```python
from build123d import *

# Parameters (mm, degrees)
SKETCH1_W           = 60
SKETCH1_H           = 40
BOSS_EXTRUDE1_DEPTH = 10
BOSS_EXTRUDE2_START = 5
SKETCH2_R           = 2.5
BOSS_EXTRUDE2_DEPTH = 5
BOSS_EXTRUDE3_START = -10
SKETCH2_3_R         = 2.5
BOSS_EXTRUDE3_DEPTH = 5
SKETCH3_W           = 34
SKETCH3_H           = 4
CUT_EXTRUDE1_DEPTH  = 124.434192994


with BuildPart() as part:
    # Sketch1 → Boss-Extrude1 (new body)
    with BuildSketch(Plane(origin=(0, 0, 0), x_dir=(1, 0, 0), z_dir=(0, 1, 0))):
        Rectangle(SKETCH1_W, SKETCH1_H)
    extrude(amount=BOSS_EXTRUDE1_DEPTH)

    # Sketch2 → Boss-Extrude2 (add)
    with BuildSketch(Plane(origin=(0, 0, 0), x_dir=(0, 0, -1), z_dir=(1, 0, 0)).offset(BOSS_EXTRUDE2_START)):
        with BuildLine():
            Line((20, 10), (20, 100))
            ThreePointArc((20, 100), (14, 106), (8, 100))
            Line((8, 100), (-20, 10))
            Line((-20, 10), (20, 10))
        make_face()
        with Locations((14, 25)):
            Circle(SKETCH2_R, mode=Mode.SUBTRACT)
        with Locations((14, 50)):
            Circle(SKETCH2_R, mode=Mode.SUBTRACT)
        with Locations((14, 75)):
            Circle(SKETCH2_R, mode=Mode.SUBTRACT)
        with Locations((14, 100)):
            Circle(SKETCH2_R, mode=Mode.SUBTRACT)
    extrude(amount=BOSS_EXTRUDE2_DEPTH)

    # Sketch2<3> → Boss-Extrude3 (add)
    with BuildSketch(Plane(origin=(0, 0, 0), x_dir=(0, 0, -1), z_dir=(1, 0, 0)).offset(BOSS_EXTRUDE3_START)):
        with BuildLine():
            Line((20, 10), (20, 100))
            ThreePointArc((20, 100), (14, 106), (8, 100))
            Line((8, 100), (-20, 10))
            Line((-20, 10), (20, 10))
        make_face()
        with Locations((14, 25)):
            Circle(SKETCH2_3_R, mode=Mode.SUBTRACT)
        with Locations((14, 50)):
            Circle(SKETCH2_3_R, mode=Mode.SUBTRACT)
        with Locations((14, 75)):
            Circle(SKETCH2_3_R, mode=Mode.SUBTRACT)
        with Locations((14, 100)):
            Circle(SKETCH2_3_R, mode=Mode.SUBTRACT)
    extrude(amount=BOSS_EXTRUDE3_DEPTH)

    # Sketch3 → Cut-Extrude1 (cut, through all)
    with BuildSketch(Plane.ZY.offset(30)):
        with Locations((0, 5)):
            Rectangle(SKETCH3_W, SKETCH3_H)
    extrude(amount=-CUT_EXTRUDE1_DEPTH, mode=Mode.SUBTRACT)


solid = part.part
```
The model under review builds one solid part; all positions refer to its coordinate system, in mm. A direction names the side the tool comes from. Round coordinates to 2 decimals unless told otherwise and drop trailing zeros. Order: outer loops, then holes, each group sorted by start corner. A loop starts at its lowest first (then second) coordinate and runs counter-clockwise, first axis right, second up. Notation, with made-up numbers: M -20,17 L -3,17 A22 ccw -3,44 Z; hole C 57.25,-30 d5. An arc over 180 degrees is marked long. Use a Markdown table: item, result.
1) Consider section A-A (y = 14.5). Write out the cut boundary in (x, z), then the cut area to 3 significant figures.
Report:
| item | result |
|---|---|
| outline | M -10,-20 L -5,-20 L -5,18.6 L -10,18.6 Z; M 5,-20 L 10,-20 L 10,18.6 L 5,18.6 Z |
| area | 386 mm^2 |
2) Consider section B-B (x = 7.5). Write out the cut boundary in (y, z).
Report:
| item | result |
|---|---|
| outline | M 0,-20 L 100,-20 A6 ccw 100,-8 L 10,20 L 0,20 Z; hole M 3,-17 L 7,-17 L 7,17 L 3,17 Z; hole C 25,-14 d5; hole C 50,-14 d5; hole C 75,-14 d5; hole C 100,-14 d5 |
3) Draft analysis for pull direction Z (two halves, no side actions). For faces 4 (the face through (0, 5, 17)), 5 (the face through (0, 10, 0)), 6 (the face through (7, 106, -14)), 7 (the face through (0, 5, -17)), state which applies: released by +Z, released by -Z, zero draft, split by the parting line, or undercut.
Report:
| item | result |
|---|---|
| face 4 | undercut |
| face 5 | zero draft |
| face 6 | split by the parting line |
| face 7 | undercut |
4) Consider section C-C (z = -10). Write out the cut boundary in (x, y).
Report:
| item | result |
|---|---|
| outline | M -30,0 L 30,0 L 30,3 L -30,3 Z; M -30,7 L 30,7 L 30,10 L 10,10 L 10,104.47 L 5,104.47 L 5,10 L -5,10 L -5,104.47 L -10,104.47 L -10,10 L -30,10 Z |
5) Insertion check: pin 1 (6.5 mm diameter, centred on y = 100, z = -14, fed in from +X); pin 2 (3 mm diameter, centred on x = -2.5, z = -5.5, fed in from +Y); pin 3 (1.5 mm diameter, centred on y = 12, z = -14.5, fed in from -X). Each pin has a flat end and moves straight along its axis. Give the tip position at first contact, or say it passes through.
Report:
| item | result |
|---|---|
| pin 1 | x = 10 |
| pin 2 | y = 10 |
| pin 3 | x = -10 |
6) Consider section D-D (x = 25). Write out the cut boundary in (y, z), then the cut area to 3 significant figures.
Report:
| item | result |
|---|---|
| outline | M 0,-20 L 10,-20 L 10,20 L 0,20 Z; hole M 3,-17 L 7,-17 L 7,17 L 3,17 Z |
| area | 264 mm^2 |
7) Wall thickness on line 1 along Y through (x, z) = (8.9, -14); line 2 along X through (y, z) = (49, -3); line 3 along Y through (x, z) = (-24, 15.5): over which ranges is each line inside the solid? List them lowest first. Write a range as [from, to].
Report:
| item | result |
|---|---|
| line 1 | [0, 3], [7, 22.5], [27.5, 47.5], [52.5, 72.5], [77.5, 97.5], [102.5, 106] |
| line 2 | [-10, -5], [5, 10] |
| line 3 | [0, 3], [7, 10] |
8) Tool access review of faces 1 (the face through (-10, 48, -4)), 2 (the face through (-7.535, 55.63, 5.804)), 3 (the face through (10, 48, -4)): name each direction out of +Z, -Z, +X, -X, +Y, -Y from which nothing blocks a thin tool from reaching the whole face with its end or side.
Report:
| item | result |
|---|---|
| face 1 | +Z, -Z, -X, +Y |
| face 2 | +Z, +X, -X, +Y |
| face 3 | +Z, -Z, +X, +Y |
